Source: CAD feature listing. Evaluate the final solid. Frame: model axes, mm. A direction names the side the tool comes from. Give positions to 0.01 mm unless a question says otherwise; leave off trailing zeros. Order: outer loops, then holes, each group sorted by start corner. A loop starts at its lowest first (then second) coordinate and runs counter-clockwise, first axis right, second up. Notation, with made-up numbers: M 72,70.5 L 114,70.5 A18 ccw 114,99.5 Z; hole C 39,24.25 d11. An arc over 180 degrees is marked long. Answer as a JSON object with one key per item and string values. Group by question number.
1. Pin query (flat end, axial travel): P1, Ø5, axis at x = 7, z = 7, coming from the +Y side; P2, Ø2.5, axis at x = -15.5, z = 7.5, coming from the -Y side; P3, Ø6, axis at y = 0, z = 9.5, coming from the -X side. Return the tip coordinate at first contact, or that it passes through.
2. Material intervals for L1, parallel to X at y = -8.5, z = 6.75; L2, parallel to Z at x = 25, y = 0; L3, parallel to X at y = -23, z = 14.75, sorted ascending. Write a range as [from, to].
3. Set-up query: faces 4 (the cylindrical face through (-27.984, 0.651, 14.457)), 5 (the flat face through (3.121, 4, 9)), 6 (the flat face through (-11.879, -9, 9)). Return all of +Z, -Z, +X, -X, +Y, -Y with unobstructed straight access to the full face (end or side cutting, diameter ignored); none if empty.
4. Section query D-D (z = 3). Output: boundary loops of the cut face in (x, y), plus the area to 3 significant figures.
5. Section query B-B (z = 9.5). Output: boundary loops of the cut face in (x, y), plus the area to 3 significant figures.
6. Pull-direction query (Y, two-part tool) for faces 1 (the flat face through (-28, -27.8, 9)), 2 (the flat face through (8, -15.65, 9)), 3 (the cylindrical face through (21.226, -0.651, 14.457)); classes: +Y half, -Y half, draft (parallel to the pull), parting line (faces both ways), or undercut.
7. Section query C-C (y = -7.5). Output: boundary loops of the cut face in (x, z), plus the area to 3 significant figures.
8. Section query A-A (y = 16.5). Output: boundary loops of the cut face in (x, z), plus the area to 3 significant figures.
from build123d import *

# Parameters (mm, degrees)
F1_DEPTH = 19
F3_R     = 5
F4_DEPTH = 16
F6_R     = 5
F7_DEPTH = 16


with BuildPart() as f1:
    # F0 (on Top) → F1 (new body)
    with BuildSketch(Plane.XY):
        Polygon((3.1210286321, 23.2000579238), (-35.3789713679, 23.2000579238), (-35.3789713679, -27.7999420762), (-20.3789713679, -27.7999420762), (-20.3789713679, 9.5500578434), (-11.8789713679, 9.5500578434), (-11.8789713679, -27.7999420762), (28.6210286321, -27.7999420762), (28.6210286321, 23.2000579238), (13.6210286321, 23.2000579238), (13.6210286321, -15.6499421298), (3.1210286321, -15.6499421298), align=None)
    extrude(amount=F1_DEPTH)

    # F3 (on offset) → F4 (cut)
    with BuildSketch(Plane.YZ.offset(28.6210286321)):
        with Locations((0, 9.5)):
            Circle(F3_R)
    extrude(amount=-F4_DEPTH, mode=Mode.SUBTRACT)

    # F6 (on offset) → F7 (cut)
    with BuildSketch(Plane(origin=(-35.3789713679, 0, 0), x_dir=(0, -1, 0), z_dir=(-1, 0, 0))):
        with Locations((0, 9.5)):
            Circle(F6_R)
    extrude(amount=-F7_DEPTH, mode=Mode.SUBTRACT)


solid = f1.part
Answer sheet:
{
 "1": {"P1": "y = -15.65", "P2": "y = 9.55", "P3": "x = -11.88"},
 "2": {"L1": "[-35.38, -20.38], [-11.88, 3.12], [13.62, 28.62]", "L2": "[0, 4.5], [14.5, 19]", "L3": "[-35.38, -20.38], [-11.88, 28.62]"},
 "3": {"face 4": "-X", "face 5": "+Z, -Z, +Y", "face 6": "+Z, -Z, -Y"},
 "4": {"outline": "M -35.38,-27.8 L -20.38,-27.8 L -20.38,9.55 L -11.88,9.55 L -11.88,-27.8 L 28.62,-27.8 L 28.62,23.2 L 13.62,23.2 L 13.62,-15.65 L 3.12,-15.65 L 3.12,23.2 L -35.38,23.2 Z", "area": "2,540 mm^2"},
 "5": {"outline": "M -35.38,-27.8 L -20.38,-27.8 L -20.38,-5 L -35.38,-5 Z; M -35.38,5 L -20.38,5 L -20.38,9.55 L -11.88,9.55 L -11.88,-27.8 L 28.62,-27.8 L 28.62,-5 L 13.62,-5 L 13.62,-15.65 L 3.12,-15.65 L 3.12,23.2 L -35.38,23.2 Z; M 13.62,5 L 28.62,5 L 28.62,23.2 L 13.62,23.2 Z", "area": "2,240 mm^2"},
 "6": {"face 1": "-Y half", "face 2": "+Y half", "face 3": "undercut"},
 "7": {"outline": "M -35.38,0 L -20.38,0 L -20.38,19 L -35.38,19 Z; M -11.88,0 L 3.12,0 L 3.12,19 L -11.88,19 Z; M 13.62,0 L 28.62,0 L 28.62,19 L 13.62,19 Z", "area": "855 mm^2"},
 "8": {"outline": "M -35.38,0 L 3.12,0 L 3.12,19 L -35.38,19 Z; M 13.62,0 L 28.62,0 L 28.62,19 L 13.62,19 Z", "area": "1,020 mm^2"}
}
